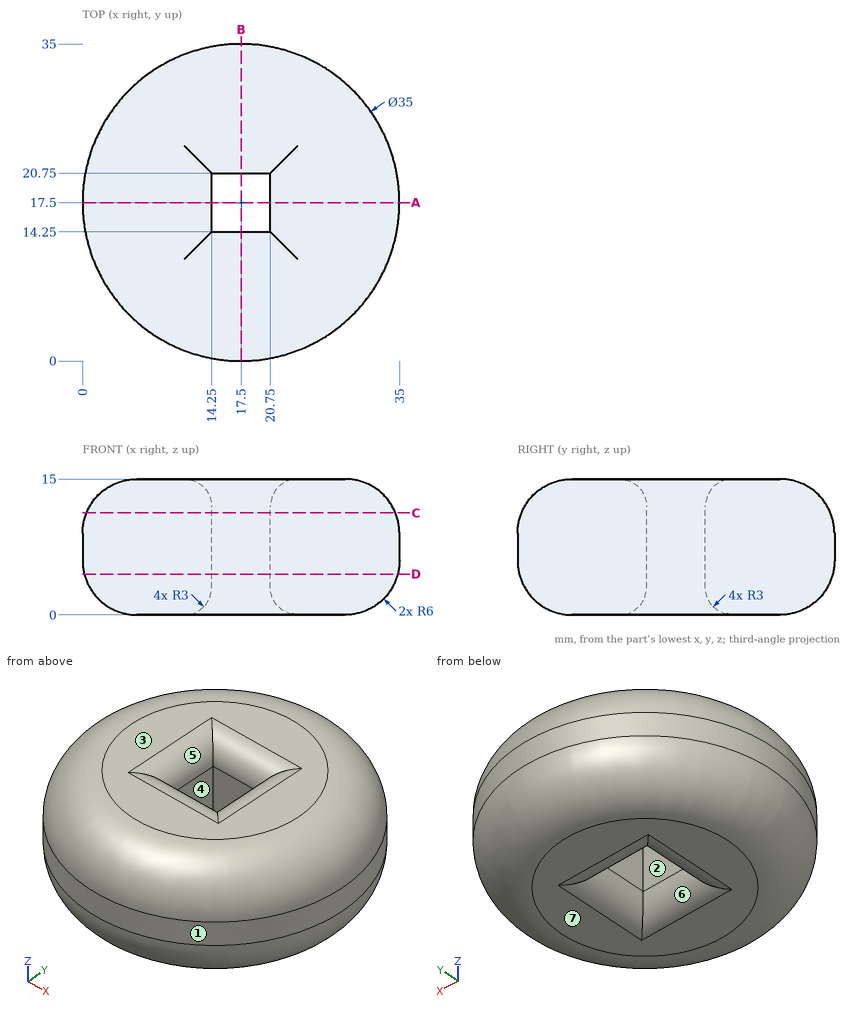
Design review of the part shown in the three views and the two pictorial views. Dimensions are in mm from the part's minimum x, y and z. A direction names the side the tool comes from. Round coordinates to 2 decimals unless told otherwise and drop trailing zeros. Order: outer loops, then holes, each group sorted by start corner. A loop starts at its lowest first (then second) coordinate and runs counter-clockwise, first axis right, second up. Notation, with made-up numbers: (16.5, 87) - (26.5, 87) arc R31 ccw to (26.5, 124) - close; hole circle Ø10 at (50.25, -20). An arc over 180 degrees is marked (long way). Answer in a Markdown table with one row per item.
(1) Mouldability with a two-part tool opening along X and no side actions: class the marked faces 1, 2 and 3 as released by +X, released by -X, zero draft, split by the parting line, or undercut.
Result set:
| item | result |
|---|---|
| face 1 | split by the parting line |
| face 2 | undercut |
| face 3 | zero draft |
(2) Take a section at D-D on z = 4.5. Write out the cut boundary in (x, y).
Result set:
| item | result |
|---|---|
| outline | circle Ø34.62 at (17.5, 17.5); hole (14.25, 14.25) - (20.75, 14.25) - (20.75, 20.75) - (14.25, 20.75) - close |
(3) For line 1 (Y direction, x = 17.5, z = 7); line 2 (Y direction, x = 29, z = 9); line 3 (X direction, y = 27, z = 10), list the stretches that pass through material, from the lowest coordinate up. Write a range as from..to.
Result set:
| item | result |
|---|---|
| line 1 | y = 0..14.25, 20.75..35 |
| line 2 | y = 4.31..30.69 |
| line 3 | x = 2.9..32.1 |
(4) Take a section at C-C on z = 11.25. Write out the cut boundary in (x, y), plus the area to 3 significant figures.
Result set:
| item | result |
|---|---|
| outline | circle Ø34.12 at (17.5, 17.5); hole (14.25, 14.25) - (20.75, 14.25) - (20.75, 20.75) - (14.25, 20.75) - close |
| area | 872 mm2 |
(5) Machinability: for the marked faces 4, 5, 6 and 7, which of the approach directions +Z, -Z, +X, -X, +Y, -Y give a long, thin tool a straight path to every point of the face, cutting with its end or side? Answer none if there is none.
Result set:
| item | result |
|---|---|
| face 4 | +Z, -Z |
| face 5 | +Z |
| face 6 | -Z |
| face 7 | -Z, +X, -X, +Y, -Y |
(6) Take a section at A-A on y = 17.5. Write out the cut boundary in (x, z), plus the area to 3 significant figures.
Result set:
| item | result |
|---|---|
| outline | (0, 6) arc R6 ccw to (6, 0) - (11.25, 0) arc R3 ccw to (14.25, 3) - (14.25, 12) arc R3 ccw to (11.25, 15) - (6, 15) arc R6 ccw to (0, 9) - close; (20.75, 3) arc R3 ccw to (23.75, 0) - (29, 0) arc R6 ccw to (35, 6) - (35, 9) arc R6 ccw to (29, 15) - (23.75, 15) arc R3 ccw to (20.75, 12) - close |
| area | 389 mm2 |
(7) Clearance check with flat-ended pins moving along their axes: P1, Ø4, axis at y = 21.5, z = 11, coming from the +X side; P2, Ø5, axis at x = 21.5, z = 12, coming from the +Y side; P3, Ø1, axis at y = 26, z = 4.5, coming from the -X side. State where each tip first meets the part, or that it passes through.
Result set:
| item | result |
|---|---|
| P1 | stops at x = 34.78 |
| P2 | stops at y = 34.74 |
| P3 | stops at x = 2.12 |
